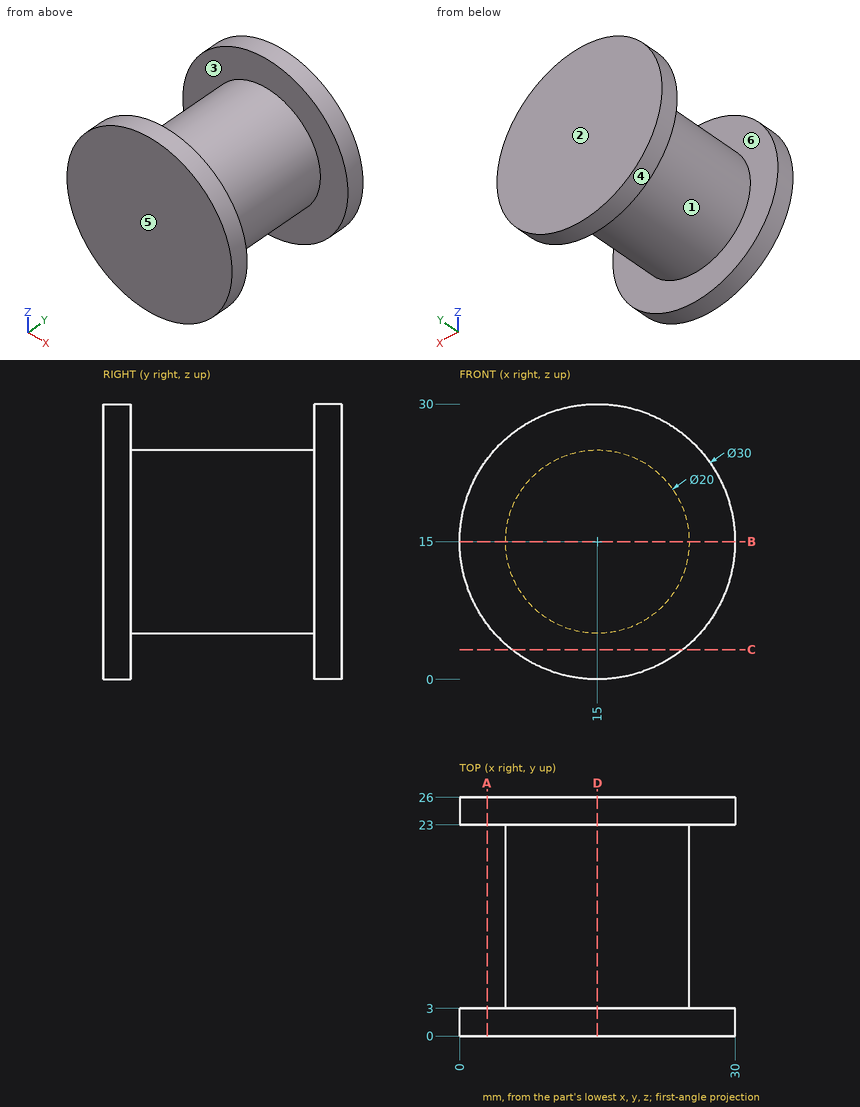
Geometry: see drawing. Coordinates: mm, zero at the bounding-box minimum. A direction names the side the tool comes from. Coordinates: 2 decimals unless noted, no trailing zeros. Order: outer loops, then holes, each group sorted by start corner. A loop starts at its lowest first (then second) coordinate and runs counter-clockwise, first axis right, second up. Notation, with made-up numbers: M 88.5,3.25 L 118.5,3.25 A32 cw 118.5,29.25 Z; hole C 50.25,4.5 d9. An arc over 180 degrees is marked long. Write item = value, one per line. Start each with the question number.
(1) Section D-D on x = 15. Output: boundary loops of the cut face in (y, z).
(2) Line query: line 1 along Y through (x, z) = (23.25, 26.75); line 2 along X through (y, z) = (9.5, 15); line 3 along Z through (x, y) = (9.5, 3.5). Output: solid intervals per line, ascending. Write a range as [from, to].
(3) Pull-direction query (Y, two-part tool) for the marked faces 1, 2, 3 and 4; classes: released by +Y, released by -Y, zero draft, split by the parting line, or undercut.
(4) Reachability of the marked faces 5 and 6 from +Z, -Z, +X, -X, +Y, -Y: full face, straight path, thin tool, end or side. Return the list, or none.
(5) Section B-B on z = 15. Output: boundary loops of the cut face in (x, y), and give its area (3 significant figures).
(6) First-contact query: P1, Ø12, axis at y = 12.5, z = 6, coming from the -X side; P2, Ø10, axis at y = 16.5, z = 10, coming from the +X side; P3, Ø1.5, axis at y = 5.5, z = 17, coming from the +X side. Flat tips, straight axial feed; report the tip coordinate or a pass-through.
(7) Section C-C on z = 3.25. Output: boundary loops of the cut face in (x, y).
(8) Section A-A on x = 3. Output: boundary loops of the cut face in (y, z), and give its area (3 significant figures).
Result set:
q1.outline = M 0,0 L 3,0 L 3,5 L 23,5 L 23,0 L 26,0 L 26,30 L 23,30 L 23,25 L 3,25 L 3,30 L 0,30 Z
q2.line_1 = [0, 3], [23, 26]
q2.line_2 = [5, 25]
q2.line_3 = [6.65, 23.35]
q3.face_1 = undercut
q3.face_2 = released by +Y
q3.face_3 = undercut
q3.face_4 = zero draft
q4.face_5 = +Z, -Z, +X, -X, -Y
q4.face_6 = none
q5.outline = M 0,0 L 30,0 L 30,3 L 25,3 L 25,23 L 30,23 L 30,26 L 0,26 L 0,23 L 5,23 L 5,3 L 0,3 Z
q5.area = 580 mm²
q6.P1 = 5.46
q6.P2 = 25
q6.P3 = 24.92
q7.outline = M 5.68,0 L 24.32,0 L 24.32,3 L 5.68,3 Z; M 5.68,23 L 24.32,23 L 24.32,26 L 5.68,26 Z
q8.outline = M 0,6 L 3,6 L 3,24 L 0,24 Z; M 23,6 L 26,6 L 26,24 L 23,24 Z
q8.area = 108 mm²
